Autodesk Inventor part; units mm, degrees
ref_plane "YZ Plane" through (0, 0, 0) normal (1, 0, 0) x (0, 1, 0)
ref_plane "XZ Plane" through (0, 0, 0) normal (0, 1, 0) x (-1, 0, 0)
ref_plane "XY Plane" through (0, 0, 0) normal (0, 0, 1) x (1, 0, 0)
sketch "Sketch1" plane through (0, 0, 0) normal (0, 1, 0) x (-1, 0, 0)
  line L0 (17.2372, 12) -> (17.2372, 28) construction
  line L1 (14.9628, 12) -> (17.2372, 12) construction
  line L2 (14.9628, 12) -> (14.9628, 28) construction
  line L3 (17.2372, 28) -> (14.9628, 28) construction
  line L4 (14.2372, 12) -> (14.2372, 28) construction
  line L5 (11.9628, 12) -> (14.2372, 12) construction
  line L6 (11.9628, 12) -> (11.9628, 28) construction
  line L7 (14.2372, 28) -> (11.9628, 28) construction
  line L8 (20.2372, 28) -> (17.9628, 28) construction
  line L9 (20.2372, 12) -> (20.2372, 28) construction
  line L10 (17.9628, 12) -> (20.2372, 12) construction
  line L11 (17.9628, 12) -> (17.9628, 28) construction
  line L12 (11.2372, 12) -> (11.2372, 28) construction
  line L13 (8.9628, 12) -> (11.2372, 12) construction
  line L14 (8.9628, 12) -> (8.9628, 28) construction
  line L15 (11.2372, 28) -> (8.9628, 28) construction
  line L16 (23.2372, 28) -> (20.9628, 28) construction
  line L17 (23.2372, 12) -> (23.2372, 28) construction
  line L18 (20.9628, 12) -> (23.2372, 12) construction
  line L19 (20.9628, 12) -> (20.9628, 28) construction
  line L20 (8.2372, 12) -> (8.2372, 28) construction
  line L21 (5.9628, 12) -> (8.2372, 12) construction
  line L22 (5.9628, 12) -> (5.9628, 28) construction
  line L23 (8.2372, 28) -> (5.9628, 28) construction
  line L24 (26.2372, 28) -> (23.9628, 28) construction
  line L25 (26.2372, 12) -> (26.2372, 28) construction
  line L26 (23.9628, 12) -> (26.2372, 12) construction
  line L27 (23.9628, 12) -> (23.9628, 28) construction
  line L28 (5.2372, 12) -> (5.2372, 28) construction
  line L29 (2.9628, 12) -> (5.2372, 12) construction
  line L30 (2.9628, 12) -> (2.9628, 28) construction
  line L31 (5.2372, 28) -> (2.9628, 28) construction
  line L32 (29.2372, 28) -> (26.9628, 28) construction
  line L33 (29.2372, 12) -> (29.2372, 28) construction
  line L34 (26.9628, 12) -> (29.2372, 12) construction
  line L35 (26.9628, 12) -> (26.9628, 28) construction
  line L36 (2.2372, 12) -> (2.2372, 28) construction
  line L37 (0, 12) -> (2.2372, 12) construction
  line L38 (0, 0) -> (0, 28)
  line L39 (45, 0) -> (0, 0)
  line L40 (45, 28) -> (45, 0)
  line L41 (43.8628, 12) -> (45, 12) construction
  line L42 (43.8628, 12) -> (43.8628, 28) construction
  line L43 (45, 28) -> (43.8628, 28) construction
  line L44 (45, 40) -> (45, 28)
  line L45 (0, 40) -> (45, 40)
  line L46 (0, 28) -> (0, 40)
  line L47 (2.2372, 28) -> (0, 28) construction
  circle A0 centre (7.05, 34) radius 2.6
  circle A1 centre (37.95, 34) radius 2.6
  circle A2 centre (37.95, 6) radius 2.6
  circle A3 centre (7.05, 6) radius 2.6
  line L48 (32.2372, 28) -> (29.9628, 28) construction
  line L49 (32.2372, 12) -> (32.2372, 28) construction
  line L50 (29.9628, 12) -> (32.2372, 12) construction
  line L51 (29.9628, 12) -> (29.9628, 28) construction
  line L52 (37.95, 6) -> (7.05, 6) construction
  line L53 (7.05, 6) -> (7.05, 34) construction
  line L54 (7.05, 34) -> (37.95, 34) construction
  line L55 (37.95, 34) -> (37.95, 6) construction
  point P0 (34.1, 12)
  dimension "d2" = 45
  dimension "d3" = 40
  dimension "d4" = 30.9
extrude "Extrusion1" add sketch "Sketch1" along normal blind 3.5
properties part number "X Axis Belt Adjustable Top"
Geometry: final body of the model. Coordinates: model frame, mm. Coordinates: 2 decimals unless noted, no trailing zeros. Order: outer loops, then holes, each group sorted by start corner. A loop starts at its lowest first (then second) coordinate and runs counter-clockwise, first axis right, second up. Notation, with made-up numbers: (-38.75, -24.5) -> (-7.75, -24.5) arc R32 cw to (-7.75, 6.5) -> close; hole circle Ø2 at (-28, -4.75). An arc over 180 degrees is marked (long way). Answer in a Markdown table with one row per item.
Item 1: Section C-C on y = 1.35. Output: boundary loops of the cut face in (x, z), plus the area to 3 significant figures.
Return value:
| item | result |
|---|---|
| outline | (-45, 0) -> (0, 0) -> (0, 40) -> (-45, 40) -> close; hole circle Ø5.2 at (-37.95, 6); hole circle Ø5.2 at (-37.95, 34); hole circle Ø5.2 at (-7.05, 6); hole circle Ø5.2 at (-7.05, 34) |
| area | 1,720 mm² |
Item 2: Section B-B on x = -7.05. Output: boundary loops of the cut face in (y, z), plus the area to 3 significant figures.
Return value:
| item | result |
|---|---|
| outline | (0, 0) -> (3.5, 0) -> (3.5, 3.4) -> (0, 3.4) -> close; (0, 8.6) -> (3.5, 8.6) -> (3.5, 31.4) -> (0, 31.4) -> close; (0, 36.6) -> (3.5, 36.6) -> (3.5, 40) -> (0, 40) -> close |
| area | 104 mm² |
Item 3: Draft query along X for faces 1 (the flat face through (-22, 0, 20)), 2 (the cylindrical face through (-6.712, 1.726, 31.422)), 3 (the flat face through (0, 2, 20)), 4 (the flat face through (-45, 2, 20)). Return one class per face: released by +X, released by -X, zero draft, split by the parting line, or undercut.
Return value:
| item | result |
|---|---|
| face 1 | zero draft |
| face 2 | undercut |
| face 3 | released by +X |
| face 4 | released by -X |
Item 4: Ray query, L1, parallel to Z at x = -7.05, y = 2.2; L2, parallel to X at y = 2.2, z = 34.5; L3, parallel to X at y = 0.5, z = 4.5. Return the intervals inside material, ascending.
Return value:
| item | result |
|---|---|
| L1 | z = 0 to 3.4, 8.6 to 31.4, 36.6 to 40 |
| L2 | x = -45 to -40.5, -35.4 to -9.6, -4.5 to 0 |
| L3 | x = -45 to -40.07, -35.83 to -9.17, -4.93 to 0 |
Item 5: Contact query for a flat-ended pin moving along its axis: P1, Ø4.5, axis at x = -37.95, z = 34, coming from the -Y side (3 decimals). Output: stop coordinate, or through.
Return value:
| item | result |
|---|---|
| P1 | passes through |
Item 6: Section A-A on z = 6. Output: boundary loops of the cut face in (x, y), plus the area to 3 significant figures.
Return value:
| item | result |
|---|---|
| outline | (-45, 0) -> (-40.55, 0) -> (-40.55, 3.5) -> (-45, 3.5) -> close; (-35.35, 0) -> (-9.65, 0) -> (-9.65, 3.5) -> (-35.35, 3.5) -> close; (-4.45, 0) -> (0, 0) -> (0, 3.5) -> (-4.45, 3.5) -> close |
| area | 121 mm² |
